```python
from build123d import *

# Parameters (mm, degrees)
F1_DEPTH = 75
F2_R     = 8
F3_R     = 5.4
F4_DEPTH = 25


with BuildPart() as f1:
    # F0 (on Front) → F1 (new body, symmetric)
    with BuildSketch(Plane.XZ):
        Polygon((0, 0), (-3, 0), (-3, -8), (86, -8), (86, 0), (6, 0), (6, 50), (0, 50), align=None)
    extrude(amount=F1_DEPTH, both=True)

    # F2
    f2_edges = [f1.edges().sort_by_distance(p)[0] for p in [
        (86, 75, -4),
        (86, -75, -4),
        (3, 75, 50),
        (3, -75, 50),
        (6, 0, 0),
    ]]
    fillet(f2_edges, radius=F2_R)

    # F3 (on Right) → F4 (cut)
    with BuildSketch(Plane.YZ):
        with Locations((-40, 34)):
            Circle(F3_R)
        with BuildLine():
            ThreePointArc((45.4, 34), (40, 39.4), (34.6, 34))
            ThreePointArc((34.6, 34), (40, 28.6), (45.4, 34))
        make_face()
    extrude(amount=F4_DEPTH, mode=Mode.SUBTRACT)


solid = f1.part
```
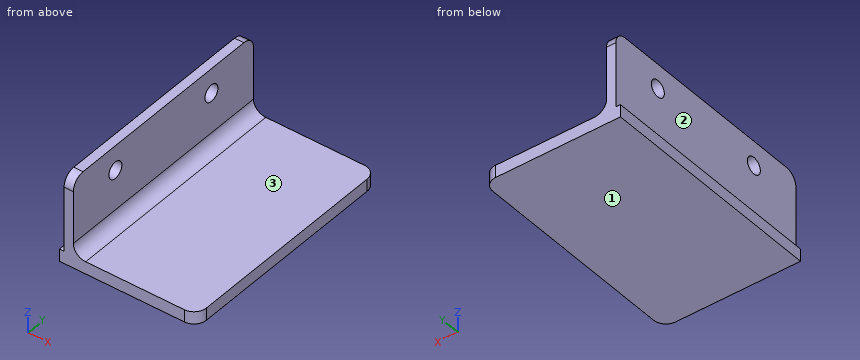
Geometry check sheet. Reference: the model listing, model coordinates, mm. Face numbers are marked on the shaded views. A direction names the side the tool comes from. Coordinates: 2 decimals unless noted, no trailing zeros. Order: outer loops, then holes, each group sorted by start corner. A loop starts at its lowest first (then second) coordinate and runs counter-clockwise, first axis right, second up.
Item 1: Scan lines: line 1 along Y through (x, z) = (2.55, 34); line 2 along Z through (x, y) = (2, -40); line 3 along Z through (x, y) = (33, 0.5). Record each from-to range of solid material in increasing order.
Item 2: Tool access check on the marked faces 1, 2 and 3. Record the directions out of +Z, -Z, +X, -X, +Y, -Y that give a thin tool (end or side, any length) a straight path to the whole face; none if there is none.
Item 3: Section check A-A (y = -40). Enter the section's corners in (x, z).
Item 4: Section check C-C (y = 56.5). Enter the section's corners in (x, z), plus the area to 3 significant figures.
Item 5: Section check B-B (z = 34). Enter the section's corners in (x, y), plus the area to 3 significant figures.
Item 6: Depth check by flat-ended pin: pin 1 (1.5 mm diameter, centred on x = -1, y = 17, fed in from +Z); pin 2 (3 mm diameter, centred on x = 9, y = 41, fed in from +Z); pin 3 (12.5 mm diameter, centred on y = 40, z = 34, fed in from -X). Enter the tip coordinate at first touch or a pass-through.
Item 7: Section check D-D (x = 54.5). Enter the section's corners in (y, z), plus the area to 3 significant figures.
Check sheet entries:
1. line 1: y = -75 to -45.4, -34.6 to 34.6, 45.4 to 75
1. line 2: z = -8 to 28.6, 39.4 to 50
1. line 3: z = -8 to 0
2. face 1: -Z, +X, -X, +Y, -Y
2. face 2: +Z, -X, +Y, -Y
2. face 3: +Z, +X, +Y, -Y
3. outline: (-3, -8) - (86, -8) - (86, 0) - (14, 0) arc R8 cw to (6, 8) - (6, 28.6) - (0, 28.6) - (0, 0) - (-3, 0) - close; (0, 39.4) - (6, 39.4) - (6, 50) - (0, 50) - close
4. outline: (-3, -8) - (86, -8) - (86, 0) - (14, 0) arc R8 cw to (6, 8) - (6, 50) - (0, 50) - (0, 0) - (-3, 0) - close
4. area: 1,030 mm2
5. outline: (0, -75) - (6, -75) - (6, -45.4) - (0, -45.4) - close; (0, -34.6) - (6, -34.6) - (6, 34.6) - (0, 34.6) - close; (0, 45.4) - (6, 45.4) - (6, 75) - (0, 75) - close
5. area: 770 mm2
6. pin 1: stops at z = 0
6. pin 2: stops at z = 3.34
6. pin 3: stops at x = 0
7. outline: (-75, -8) - (75, -8) - (75, 0) - (-75, 0) - close
7. area: 1,200 mm2
